from build123d import *

# Parameters (mm, degrees)
SKETCH_2_W          = 38.6
SKETCH_2_H          = 9.4
EXTRUDE_1_DEPTH     = 1
SKETCH_3_W          = 1
SKETCH_3_H          = 9.4
EXTRUDE_2_DEPTH     = 28.5
SKETCH_4_R          = 12.5
EXTRUDE_3_DEPTH     = 1
CUT_EXTRUDE_1_DEPTH = 37.619530308
CUT_EXTRUDE_2_DEPTH = 51.164329957
SKETCH_7_R          = 1
CUT_EXTRUDE_3_DEPTH = 51.164329957
FILLET_1_R          = 3


with BuildPart() as part:
    # 草图2 → 凸台-拉伸1 (new body)
    with BuildSketch(Plane(origin=(0, 0, 0), x_dir=(1, 0, 0), z_dir=(0, 1, 0))):
        Rectangle(SKETCH_2_W, SKETCH_2_H)
    extrude(amount=EXTRUDE_1_DEPTH)

    # 草图3 → 凸台-拉伸2 (add)
    with BuildSketch(Plane(origin=(0, 1, 0), x_dir=(1, 0, 0), z_dir=(0, 1, 0))):
        with Locations((-18.8, 0)):
            Rectangle(SKETCH_3_W, SKETCH_3_H)
        with Locations((18.8, 0)):
            Rectangle(SKETCH_3_W, SKETCH_3_H)
    extrude(amount=EXTRUDE_2_DEPTH)

    # 草图4 → 凸台-拉伸3 (add)
    with BuildSketch(Plane(origin=(0, 1, 0), x_dir=(1, 0, 0), z_dir=(0, 1, 0))):
        Circle(SKETCH_4_R)
        with BuildLine():
            ThreePointArc((5, -8.660254038), (0, -10), (-5, -8.660254038))
            ThreePointArc((-5, -8.660254038), (-5.549038106, -6.611215932), (-3.5, -6.062177826))
            ThreePointArc((-3.5, -6.062177826), (0, -7), (3.5, -6.062177826))
            ThreePointArc((3.5, -6.062177826), (5.549038106, -6.611215932), (5, -8.660254038))
        make_face(mode=Mode.SUBTRACT)
        with BuildLine():
            ThreePointArc((5, 8.660254038), (0, 10), (-5, 8.660254038))
            ThreePointArc((-5, 8.660254038), (-5.549038106, 6.611215932), (-3.5, 6.062177826))
            ThreePointArc((-3.5, 6.062177826), (0, 7), (3.5, 6.062177826))
            ThreePointArc((3.5, 6.062177826), (5.549038106, 6.611215932), (5, 8.660254038))
        make_face(mode=Mode.SUBTRACT)
    extrude(amount=-EXTRUDE_3_DEPTH)

    # 草图5 → 切除-拉伸1 (cut, through all)
    with BuildSketch(Plane(origin=(0, 1, 0), x_dir=(1, 0, 0), z_dir=(0, 1, 0))):
        with BuildLine():
            Line((13.7, -1.5), (7.7, -1.5))
            ThreePointArc((7.7, -1.5), (6.2, 0), (7.7, 1.5))
            Line((7.7, 1.5), (13.7, 1.5))
            ThreePointArc((13.7, 1.5), (15.2, 0), (13.7, -1.5))
        make_face()
        with BuildLine():
            Line((-13.7, -1.5), (-7.7, -1.5))
            ThreePointArc((-7.7, -1.5), (-6.2, 0), (-7.7, 1.5))
            Line((-7.7, 1.5), (-13.7, 1.5))
            ThreePointArc((-13.7, 1.5), (-15.2, 0), (-13.7, -1.5))
        make_face()
    extrude(amount=-CUT_EXTRUDE_1_DEPTH, mode=Mode.SUBTRACT)

    # 草图6 → 切除-拉伸2 (cut, through all)
    with BuildSketch(Plane(origin=(19.3, 0, 0), x_dir=(0, 0, -1), z_dir=(1, 0, 0))):
        Polygon((-4.7, 29.5), (-4.7, 1), (-2.7, 29.5), align=None)
        Polygon((4.7, 1), (2.7, 29.5), (4.7, 29.5), align=None)
    extrude(amount=-CUT_EXTRUDE_2_DEPTH, mode=Mode.SUBTRACT)

    # 草图7 → 切除-拉伸3 (cut, through all)
    with BuildSketch(Plane(origin=(19.3, 0, 0), x_dir=(0, 0, -1), z_dir=(1, 0, 0))):
        with Locations((0, 27.5)):
            Circle(SKETCH_7_R)
    extrude(amount=-CUT_EXTRUDE_3_DEPTH, mode=Mode.SUBTRACT)

    # 圆角1
    # the kernel refuses this fillet: 3 mm, written as the material it takes off along each edge
    with BuildSketch(Plane(origin=(-11.307871249, 29.5, -2.7), x_dir=(0, -0.9975467611004155, -0.0700032814807308), z_dir=(-1, 0, 0))) as fillet_1_piece_1:
        with BuildLine():
            CenterArc((FILLET_1_R * 0.932283833485, FILLET_1_R), FILLET_1_R, 184.014175695, 85.985824305)
            Line((-FILLET_1_R * 0.0652629276154, FILLET_1_R * 0.929996718519), (0, 0))
            Line((0, 0), (FILLET_1_R * 0.932283833485, 0))
        make_face()
    extrude(amount=14.984257502, mode=Mode.SUBTRACT)
    with BuildSketch(Plane(origin=(-11.307871249, 29.5, 2.7), x_dir=(0, -0.9975467611004155, 0.0700032814807308), z_dir=(-1, 0, 0)), Plane(origin=(26.292128751, 29.5, -2.7), x_dir=(0, 0, 1), z_dir=(-1, 0, 0)), Plane(origin=(26.292128751, 29.5, 2.7), x_dir=(0, -0.9975467611004155, 0.0700032814807308), z_dir=(-1, 0, 0))) as fillet_1_piece_2:
        with BuildLine():
            CenterArc((FILLET_1_R * 0.932283833485, -FILLET_1_R), FILLET_1_R, 90, 85.985824305)
            Line((-FILLET_1_R * 0.0652629276154, -FILLET_1_R * 0.929996718519), (0, 0))
            Line((0, 0), (FILLET_1_R * 0.932283833485, 0))
        make_face()
    extrude(amount=14.984257502, mode=Mode.SUBTRACT)


solid = part.part
The listing builds one solid part. Answer for the finished solid, in the listing's coordinates (mm). A direction names the side the tool comes from. Round coordinates to 2 decimals unless told otherwise and drop trailing zeros. Order: outer loops, then holes, each group sorted by start corner. A loop starts at its lowest first (then second) coordinate and runs counter-clockwise, first axis right, second up. Notation, with made-up numbers: (79.25, -9.75) -> (131.25, -9.75) arc R19 ccw to (131.25, -2.75) -> close; hole circle Ø6 at (-13.5, 70). An arc over 180 degrees is marked (long way). One line per item, written item: value.
Item 1: Find section D-D, the plane y = 27.5. Give the vertices of the cut face in (x, z).
Taken from the geometry:
outline: (-19.3, -2.73) -> (-18.3, -2.73) -> (-18.3, -1) -> (-19.3, -1) -> close; (-19.3, 1) -> (-18.3, 1) -> (-18.3, 2.73) -> (-19.3, 2.73) -> close; (18.3, -2.73) -> (19.3, -2.73) -> (19.3, -1) -> (18.3, -1) -> close; (18.3, 1) -> (19.3, 1) -> (19.3, 2.73) -> (18.3, 2.73) -> close
Item 2: Given P1, Ø1.5, axis at x = 3.5, z = -6, coming from the +Y side; P2, Ø1.8, axis at y = 27.5, z = 0, coming from the +X side (3 decimals); P3, Ø0.5, axis at x = -16, y = 0.5, coming from the -Z side; P4, Ø0.8, axis at x = 11.5, y = 0.5, coming from the -Z side, each flat-ended and moving along its own axis, determine where each tip first touches the part or whether it passes through.
Taken from the geometry:
P1: stops at y = 1
P2: passes through
P3: stops at z = -4.7
P4: stops at z = -5.75
Item 3: For a pull along Z with two mould halves and no side action, classify faces 1 (the flat face through (-15.5, 0.5, 4.7)), 2 (the cylindrical face through (-5.565, 0.507, 6.64)), 3 (the flat face through (18.3, 12, 0)) as released by +Z, released by -Z, zero draft, split by the parting line, or undercut.
Taken from the geometry:
face 1: released by +Z
face 2: undercut
face 3: zero draft
Item 4: For faces 4 (the flat face through (0, 1, 0)), 5 (the cylindrical face through (0.1, 0.5, -10)), 6 (the flat face through (15.4, 0.5, 4.7)), determine the directions among +Z, -Z, +X, -X, +Y, -Y from which every point of the face is accessible in a straight line to the end or side of a thin tool.
Taken from the geometry:
face 4: +Z, -Z, +Y
face 5: +Y, -Y
face 6: +Z, +X, +Y, -Y
Item 5: Straight lines are drawn through the part: L1, parallel to Y at x = -18.8, z = 0; L2, parallel to X at y = 13, z = -2; L3, parallel to Y at x = 1, z = -4.75. For each, find the intervals that lie inside material, in ascending order.
Taken from the geometry:
L1: y = 0 to 26.5, 28.5 to 29.5
L2: x = -19.3 to -18.3, 18.3 to 19.3
L3: y = 0 to 1
Item 6: Find section A-A, the plane y = 13. Give the vertices of the cut face in (x, z).
Taken from the geometry:
outline: (-19.3, -3.86) -> (-18.3, -3.86) -> (-18.3, 3.86) -> (-19.3, 3.86) -> close; (18.3, -3.86) -> (19.3, -3.86) -> (19.3, 3.86) -> (18.3, 3.86) -> close
Item 7: Find section B-B, the plane x = -4. Give the vertices of the cut face in (y, z).
Taken from the geometry:
outline: (0, -11.84) -> (1, -11.84) -> (1, -9.17) -> (0, -9.17) -> close; (0, -5.88) -> (1, -5.88) -> (1, 5.88) -> (0, 5.88) -> close; (0, 9.17) -> (1, 9.17) -> (1, 11.84) -> (0, 11.84) -> close
Item 8: Find section C-C, the plane z = -0.5. Give the vertices of the cut face in (x, y).
Taken from the geometry:
outline: (-19.3, 0) -> (-15.11, 0) -> (-15.11, 1) -> (-18.3, 1) -> (-18.3, 26.63) -> (-19.3, 26.63) -> close; (-19.3, 28.37) -> (-18.3, 28.37) -> (-18.3, 29.44) -> (-19.3, 29.44) -> close; (-6.29, 0) -> (6.29, 0) -> (6.29, 1) -> (-6.29, 1) -> close; (15.11, 0) -> (19.3, 0) -> (19.3, 26.63) -> (18.3, 26.63) -> (18.3, 1) -> (15.11, 1) -> close; (18.3, 28.37) -> (19.3, 28.37) -> (19.3, 29.44) -> (18.3, 29.44) -> close
